Design review of the part built by this model. Coordinates are the model's own, in mm. Round coordinates to 2 decimals unless told otherwise and drop trailing zeros. Order: outer loops, then holes, each group sorted by start corner. A loop starts at its lowest first (then second) coordinate and runs counter-clockwise, first axis right, second up.
from build123d import *

# Parameters (mm, degrees)
BOSS_EXTRUDE1_DEPTH       = 6
FILLET1_R                 = 10
F_4_0MM_DOWEL_HOLE1_D     = 4
F_4_0MM_DOWEL_HOLE1_DEPTH = 98.31
F_4_0MM_DOWEL_HOLE1_TIP   = 1.201721238


with BuildPart() as part:
    # Sketch1 → Boss-Extrude1 (new body)
    with BuildSketch(Plane(origin=(0, 0, 0), x_dir=(1, 0, 0), z_dir=(0, 1, 0))):
        Polygon((50, 50), (60, 50), (60, -50), (50, -50), (-50, -50), (-50, 50), align=None)
    extrude(amount=BOSS_EXTRUDE1_DEPTH)

    # Fillet1
    fillet1_edges = [part.edges().sort_by_distance(p)[0] for p in [
        (-50, 3, -50),
        (-50, 3, 50),
    ]]
    fillet(fillet1_edges, radius=FILLET1_R)

    # Ø4.0mm Dowel Hole1
    with Locations(Plane(origin=(0, 6, 0), x_dir=(1, 0, 0), z_dir=(0, 1, 0))):
        with Locations((-28, 36.483109463), (28.463106056, 36.483109463), (-28, -36.483109463), (28.463106056, -36.483109463)):
            Hole(F_4_0MM_DOWEL_HOLE1_D / 2, depth=F_4_0MM_DOWEL_HOLE1_DEPTH)
            with Locations((0, 0, -(F_4_0MM_DOWEL_HOLE1_DEPTH + F_4_0MM_DOWEL_HOLE1_TIP / 2))):  # 118° drill point
                Cone(0, F_4_0MM_DOWEL_HOLE1_D / 2, F_4_0MM_DOWEL_HOLE1_TIP, mode=Mode.SUBTRACT)


solid = part.part
1) The part is to be moulded in two halves that separate along Z. For faces 1 (the face through (6, 6, -1)), 2 (the face through (-46.99, 3.04, -47.15)), 3 (the face through (27.54, 2.958, 38.257)), say which applies: released by +Z, released by -Z, zero draft, split by the parting line, or undercut.
Results:
face 1: zero draft
face 2: released by -Z
face 3: undercut
2) Clearance check with a flat-ended pin moving along its axis: P1, Ø3.5, axis at x = -28, z = -36.48, coming from the -Y side. State where the tip first meets the part, or that it passes through.
Results:
P1: passes through
3) Take a section at A-A on x = -28. Give the boundary of the cut face in (y, z), plus the area to 3 significant figures.
Results:
outline: (0, -50) - (6, -50) - (6, -38.48) - (0, -38.48) - close; (0, -34.48) - (6, -34.48) - (6, 34.48) - (0, 34.48) - close; (0, 38.48) - (6, 38.48) - (6, 50) - (0, 50) - close
area: 552 mm2
4) To check wall thickness, follow line 1 along Z through (x, y) = (-28, 3.5); line 2 along X through (y, z) = (5.3, 36.5); line 3 along X through (y, z) = (4.4, -36). State the ranges of each line that lie inside material, in increasing order.
Results:
line 1: z = -50 to -38.48, -34.48 to 34.48, 38.48 to 50
line 2: x = -50 to -30, -26 to 26.46, 30.46 to 60
line 3: x = -50 to -29.94, -26.06 to 26.52, 30.4 to 60
